For this review, use the dimensioned drawing (mm, ordinates from the lowest corner) and the shaded views. A direction names the side the tool comes from. Give positions to 0.01 mm unless a question says otherwise; leave off trailing zeros. Write each loop counter-clockwise with the first axis right and the second up, starting at its lowest first coordinate (ties: lowest second). Pieces come first, ordered by that corner, then holes. Notation, with made-up numbers: (32.5, -27.75) -> (85.5, -27.75) arc R9 cw to (85.5, -16.75) -> close; hole circle Ø8 at (-4, 20.5). An arc over 180 degrees is marked (long way). Answer as CSV lines item,"result".
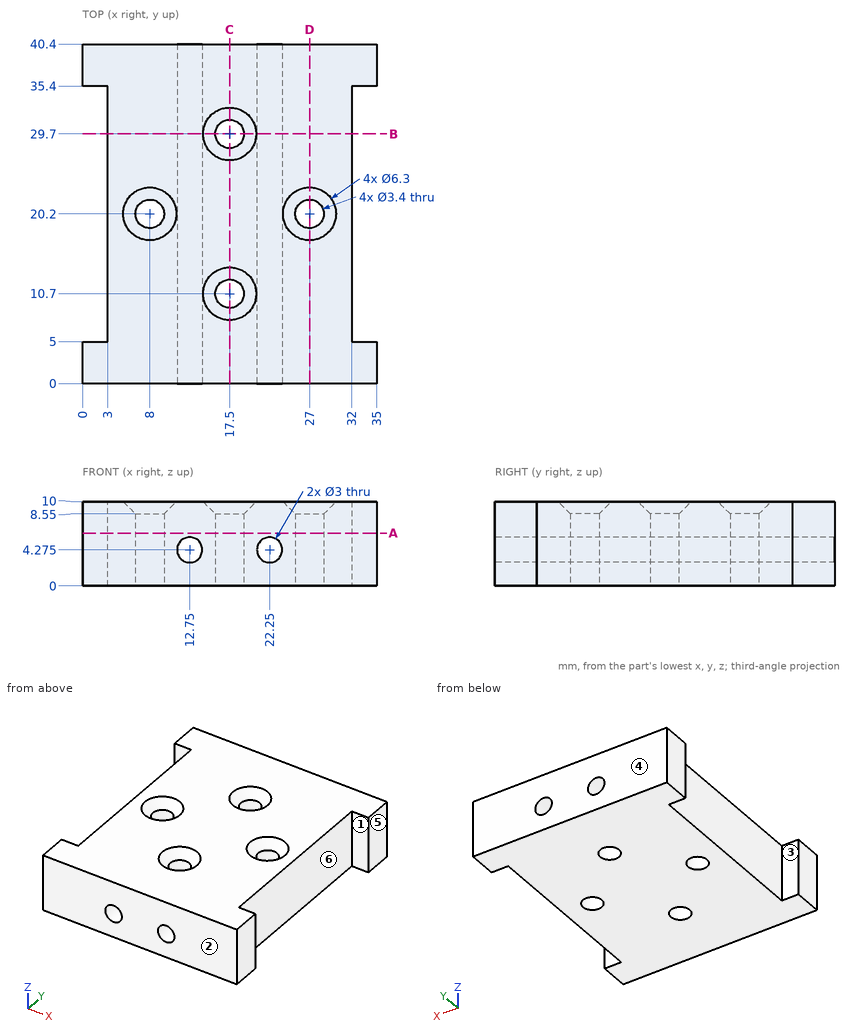
Q1. For the marked faces 1, 2 and 3, list the 3-axis set-ups (+Z, -Z, +X, -X, +Y, -Y) from which the entire face can be reached by the end or side of a thin tool; tool diameter is ignored.
Answer block:
face 1,"+Z, -Z, +X"
face 2,"+Z, -Z, +X, -X, -Y"
face 3,"+Z, -Z, -X"
Q2. Clearance check with flat-ended pins moving along their axes: pin 1 (5.5 mm diameter, centred on x = 17.5, y = 10.7, fed in from +Z); pin 2 (2 mm diameter, centred on x = 8, y = 20.2, fed in from -Z); pin 3 (3 mm diameter, centred on y = 27.5, z = 3.5, fed in from +X); pin 4 (5 mm diameter, centred on y = 17.5, z = 6, fed in from -X). State where each tip first meets the part, or that it passes through.
Answer block:
pin 1,"stops at z = 9.6"
pin 2,"passes through"
pin 3,"stops at x = 32"
pin 4,"stops at x = 3"
Q3. Add section A-A (z = 6.25). Write out the cut boundary in (x, y), plus the area to 3 significant figures.
Answer block:
outline,"(0, 0) -> (35, 0) -> (35, 5) -> (32, 5) -> (32, 35.4) -> (35, 35.4) -> (35, 40.4) -> (0, 40.4) -> (0, 35.4) -> (3, 35.4) -> (3, 5) -> (0, 5) -> close; hole circle Ø3.4 at (8, 20.2); hole circle Ø3.4 at (17.5, 10.7); hole circle Ø3.4 at (17.5, 29.7); hole circle Ø3.4 at (27, 20.2)"
area,"1,200 mm2"
Q4. Add section D-D (x = 27). Write out the cut boundary in (y, z).
Answer block:
outline,"(0, 0) -> (18.5, 0) -> (18.5, 8.55) -> (17.05, 10) -> (0, 10) -> close; (21.9, 0) -> (40.4, 0) -> (40.4, 10) -> (23.35, 10) -> (21.9, 8.55) -> close"
Q5. Add section B-B (y = 29.7). Write out the cut boundary in (x, z) (3 decimals).
Answer block:
outline,"(3, 0) -> (15.8, 0) -> (15.8, 8.55) -> (14.35, 10) -> (3, 10) -> close; (19.2, 0) -> (32, 0) -> (32, 10) -> (20.65, 10) -> (19.2, 8.55) -> close; hole circle Ø3 at (12.75, 4.275); hole circle Ø3 at (22.25, 4.275)"
Q6. Draft analysis for pull direction Y (two halves, no side actions). For the marked faces 4, 5 and 6, state which applies: released by +Y, released by -Y, zero draft, split by the parting line, or undercut.
Answer block:
face 4,"released by +Y"
face 5,"zero draft"
face 6,"undercut"
Q7. To check wall thickness, follow probe 1 along Y at (x, z) = (17.5, 5); probe 2 along Y at (x, z) = (2, 3.75); probe 3 along Z at (x, y) = (12.75, 31.5) (3 decimals). State the ranges of each line that lie inside material, in increasing order. Write a range as [from, to].
Answer block:
probe 1,"y = [0, 9], [12.4, 28], [31.4, 40.4]"
probe 2,"y = [0, 5], [35.4, 40.4]"
probe 3,"z = [0, 2.775], [5.775, 10]"
Q8. Add section C-C (x = 17.5). Write out the cut boundary in (y, z).
Answer block:
outline,"(0, 0) -> (9, 0) -> (9, 8.55) -> (7.55, 10) -> (0, 10) -> close; (12.4, 0) -> (28, 0) -> (28, 8.55) -> (26.55, 10) -> (13.85, 10) -> (12.4, 8.55) -> close; (31.4, 0) -> (40.4, 0) -> (40.4, 10) -> (32.85, 10) -> (31.4, 8.55) -> close"
